```python
from build123d import *

# Parameters (mm, degrees)
SKETCH_1_W          = 7
SKETCH_1_H          = 7
EXTRUDE_1_DEPTH     = 107
FILLET_1_R          = 3.5
SKETCH_5_R          = 1.55
CUT_EXTRUDE_2_DEPTH = 108.285833175
SKETCH_6_W          = 7
SKETCH_6_H          = 4
EXTRUDE_2_DEPTH     = 7
FILLET_2_R          = 3.5
SKETCH_7_R          = 1.5
CUT_EXTRUDE_3_DEPTH = 104.592953428
FILLET_3_R          = 3.5
FILLET_4_R          = 0.8
FILLET_5_R          = 0.8


# Some blends are built 0.0001 mm under size
with BuildPart() as part:
    # 草图1 → 凸台-拉伸1 (new body)
    with BuildSketch(Plane.XY):
        Rectangle(SKETCH_1_W, SKETCH_1_H)
    extrude(amount=EXTRUDE_1_DEPTH)

    # 圆角1
    fillet_1_edges = [part.edges().sort_by_distance(p)[0] for p in [
        (0, -3.5, 107),
    ]]
    fillet(fillet_1_edges, radius=FILLET_1_R)

    # 草图5 → 切除-拉伸2 (cut, through all)
    with BuildSketch(Plane(origin=(3.5, 0, 0), x_dir=(0, 0, -1), z_dir=(1, 0, 0))):
        with Locations(Location((-103.5, 0, 0), (0, 0, 90))):
            Circle(SKETCH_5_R)
    extrude(amount=-CUT_EXTRUDE_2_DEPTH, mode=Mode.SUBTRACT)

    # 草图6 → 凸台-拉伸2 (add)
    with BuildSketch(Plane(origin=(0, 3.5, 0), x_dir=(1, 0, 0), z_dir=(0, 1, 0))):
        with Locations((0, -105)):
            Rectangle(SKETCH_6_W, SKETCH_6_H)
    extrude(amount=EXTRUDE_2_DEPTH)

    # 圆角2
    fillet_2_edges = [part.edges().sort_by_distance(p)[0] for p in [
        (3.5, 10.5, 105),
        (-3.5, 10.5, 105),
    ]]
    fillet(fillet_2_edges, radius=FILLET_2_R - 0.0001)  # a hair under: the kernel refuses the full size

    # 草图7 → 切除-拉伸3 (cut, through all)
    with BuildSketch(Plane(origin=(0, 0, 103), x_dir=(-1, 0, 0), z_dir=(0, 0, -1))):
        with Locations((0, 7)):
            Circle(SKETCH_7_R)
    extrude(amount=-CUT_EXTRUDE_3_DEPTH, mode=Mode.SUBTRACT)

    # 圆角3
    # the kernel refuses this fillet: 3.5 mm, written as the material it adds along each edge
    with BuildSketch(Plane(origin=(-3.5, 3.5, 103), x_dir=(0, 1, 0), z_dir=(1, 0, 0))) as fillet_3_piece_1_section:
        with BuildLine():
            CenterArc((FILLET_3_R, -FILLET_3_R), FILLET_3_R, 90, 90)
            Line((0, -FILLET_3_R), (0, 0))
            Line((0, 0), (FILLET_3_R, 0))
        make_face()
    fillet_3_piece_1 = extrude(amount=7, mode=Mode.PRIVATE)
    fillet_3_piece_1 = fillet_3_piece_1 - Plane(origin=(0, 7, 102.188347769), x_dir=(-1, 0, 0), z_dir=(0, 0, -1)) * Cylinder(1.5, 28, mode=Mode.PRIVATE)
    add(fillet_3_piece_1)

    # 圆角4
    fillet_4_edges = [part.edges().sort_by_distance(p)[0] for p in [
        (-2.474903023, 9.474903023, 103),
        (2.474903023, 9.474903023, 103),
        (3.5, 3.5, 49.75),
        (-3.5, 3.5, 49.75),
        (-3.5, 4.525126266, 101.974873734),
        (3.5, 4.525126266, 101.974873734),
    ]]
    fillet(fillet_4_edges, radius=FILLET_4_R)

    # 圆角5
    fillet_5_edges = [part.edges().sort_by_distance(p)[0] for p in [
        (3.5, 3.50005, 107),
        (3.5, -3.5, 51.75),
        (3.5, -2.474873734, 105.974873734),
        (-3.5, -3.5, 51.75),
        (-3.5, -2.474873734, 105.974873734),
        (-3.5, 3.50005, 107),
        (-2.474903023, 9.474903023, 107),
        (2.474903023, 9.474903023, 107),
    ]]
    fillet(fillet_5_edges, radius=FILLET_5_R)


solid = part.part
```
The listing builds one solid part. Answer for the finished solid, in the listing's coordinates (mm). A direction names the side the tool comes from. Give positions to 0.01 mm unless a question says otherwise; leave off trailing zeros. Loops run counter-clockwise (first coordinate to the right, second up) from the corner with the lowest first, then second, coordinate; pieces in that order, holes last. Notation, with made-up numbers: M -32.5,12.5 L -16.5,12.5 A13 ccw -16.5,19.5 Z; hole C 5,23 d8. An arc over 180 degrees is marked long. One line per item, written item: value.
1. Each of these flat-tipped pins is pushed along its axis until it touches: P1, Ø1.3, axis at x = -0.5, y = 8, coming from the -Z side; P2, Ø5, axis at y = 7.5, z = 60, coming from the -X side; P3, Ø3, axis at x = 1.5, z = 63, coming from the +Y side. Where does it stop, or does it pass through?
Found:
P1: z = 103
P2: through
P3: y = 3.5
2. For faces 1 (the face through (0, 3.5, 49)), 2 (the face through (0.04, -2.5, 105.95)), determine the directions among +Z, -Z, +X, -X, +Y, -Y from which every point of the face is accessible in a straight line to the end or side of a thin tool.
Found:
face 1: -Z, +X, -X, +Y
face 2: +Z, +X, -X, -Y
3. Section A-A on z = 20 is taken. Determine the outline of the cut face in (x, y), plus the area to 3 significant figures.
Found:
outline: M -3.5,-2.7 A0.8 ccw -2.7,-3.5 L 2.7,-3.5 A0.8 ccw 3.5,-2.7 L 3.5,2.7 A0.8 ccw 2.7,3.5 L -2.7,3.5 A0.8 ccw -3.5,2.7 Z
area: 48.5 mm^2
4. For a pull along Z with two mould halves and no side action, classify faces 3 (the face through (-0.04, 4.55, 102)), 4 (the face through (-3.5, 0, 54)), 5 (the face through (0.049, -0.202, 105.037)) as pulls with the +Z half, pulls with the -Z half, needs draft (parallel to the pull), parting line crosses it, or undercut.
Found:
face 3: pulls with the -Z half
face 4: needs draft
face 5: undercut
5. Find the intervals of material crossed by probe 1 along X at (y, z) = (7, 104.6); probe 2 along Z at (x, y) = (2, 0); probe 3 along Y at (x, z) = (0, 103.7), in increasing order.
Found:
probe 1: -3.5 to -1.5, 1.5 to 3.5
probe 2: 0 to 101.95, 105.05 to 107
probe 3: -3.49 to -1.54, 1.54 to 5.5, 8.5 to 10.49
